Verification items for the finished model (mm, model axes). Face numbers are marked on the shaded views. Round coordinates to 2 decimals unless told otherwise and drop trailing zeros. Loops run counter-clockwise (first coordinate to the right, second up) from the corner with the lowest first, then second, coordinate; pieces in that order, holes last. Notation, with made-up numbers: (15, 18.5) -> (72, 18.5) arc R33 cw to (72, 46.5) -> close; hole circle Ø2 at (2.25, -2.5). An arc over 180 degrees is marked (long way). Write item = value, one per line.
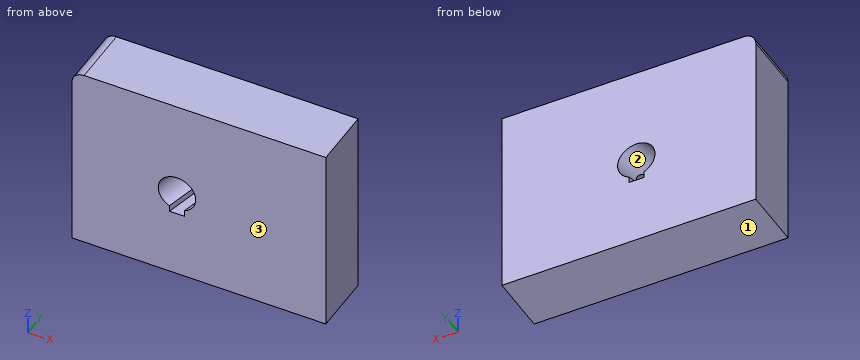
```python
from build123d import *

# Parameters (mm, degrees)
F1_DEPTH      = 25
F4_DEPTH      = 24.3161811297
F4_DEPTH_BACK = 24.3161811297
F5_R          = 4
F6_DEPTH      = 25


with BuildPart() as f1:
    # F0 (on Front) → F1 (new body)
    with BuildSketch(Plane.XZ):
        with BuildLine():
            Line((55.3635079414, 40.9526537359), (-44.2383363843, 40.9526537359))
            ThreePointArc((-44.2383363843, 40.9526537359), (-47.7738702902, 39.4881876418), (-49.2383363843, 35.9526537359))
            Line((-49.2383363843, 35.9526537359), (-49.2383363843, -37.7181139815))
            Line((-49.2383363843, -37.7181139815), (55.3635079414, -37.7181139815))
            Line((55.3635079414, -37.7181139815), (55.3635079414, 40.9526537359))
        make_face()
    extrude(amount=F1_DEPTH)

    # F3 (on 3pt) → F4 (cut, two sides)
    with BuildSketch(Plane(origin=(-2.6606007252, -11.1321497148, 0), x_dir=(-0.9726072452, 0.2324546119, 0), z_dir=(0.2324546119, 0.9726072452, 0))) as f4_sk:
        with BuildLine():
            Line((3, -9.5), (3, -6.8738635424))
            ThreePointArc((3, -6.8738635424), (0, 7.5), (-3, -6.8738635424))
            Line((-3, -6.8738635424), (-3, -9.5))
            Line((-3, -9.5), (3, -9.5))
        make_face()
    extrude(amount=-F4_DEPTH, mode=Mode.SUBTRACT)
    extrude(f4_sk.sketch, amount=F4_DEPTH_BACK, mode=Mode.SUBTRACT)

    # F5 (on Right) → F6 (cut)
    with BuildSketch(Plane.YZ):
        with Locations((-13.9910853659, 0)):
            Circle(F5_R)
    extrude(amount=F6_DEPTH, mode=Mode.SUBTRACT)


solid = f1.part
```
(1) Sectioned sample at A-A, the plane z = 0. Record the cut outline in (x, y).
Filled sheet:
outline = (-49.24, -25) -> (-13.69, -25) -> (-7.71, 0) -> (-49.24, 0) -> close; (1.74, -25) -> (55.36, -25) -> (55.36, 0) -> (7.71, 0) -> (5.32, -9.99) -> (25, -9.99) -> (25, -17.99) -> (3.41, -17.99) -> close
(2) Draft check along Z on the marked faces 1, 2 and 3. Enter one of: released by +Z, released by -Z, zero draft, split by the parting line, or undercut.
Filled sheet:
face_1 = released by -Z
face_2 = undercut
face_3 = zero draft
(3) Material ranges on probe 1 along Y at (x, z) = (18, 0); probe 2 along X at (y, z) = (-1.5, 2); probe 3 along Z at (x, y) = (-6.5, -12), recorded low to high. Write a range as from..to.
Filled sheet:
probe_1 = -25..-17.99, -9.99..0
probe_2 = -49.24..-7.79, 7.07..55.36
probe_3 = -37.72..-6.62, 6.62..40.95
